Could you check a few things on this model? Use its own coordinates, in mm. A direction names the side the tool comes from. Round coordinates to 2 decimals unless told otherwise and drop trailing zeros. Loops run counter-clockwise (first coordinate to the right, second up) from the corner with the lowest first, then second, coordinate; pieces in that order, holes last. Notation, with made-up numbers: M -25,59.25 L 25,59.25 A31 ccw 25,98.25 Z; hole C 4,23 d11. An arc over 180 degrees is marked long. Answer in a Markdown table with one row per item.
```python
from build123d import *

# Parameters (mm, degrees)
SKETCH1_W        = 50
SKETCH1_H        = 50
SKETCH1_R        = 1.5
SUPPORT_DEPTH    = 8
NORTH_START      = -25
SKETCH2_W        = 20
SKETCH2_H        = 5
NORTH_CUT_DEPTH  = 4
WEST_START       = -25
SKETCH3_W        = 20
SKETCH3_H        = 5
WEST_CUT_DEPTH   = 4
EAST_START       = 25
SKETCH3_3_W      = 20
SKETCH3_3_H      = 5
EAST_DOWEL_DEPTH = 4


with BuildPart() as part:
    # Sketch1 → Support (new body)
    with BuildSketch(Plane(origin=(0, 0, 0), x_dir=(1, 0, 0), z_dir=(0, 1, 0))):
        Rectangle(SKETCH1_W, SKETCH1_H)
        with Locations(Location((-21, -21, 0), (0, 0, 270))):
            Circle(SKETCH1_R, mode=Mode.SUBTRACT)
        with Locations(Location((21, -21, 0), (0, 0, 270))):
            Circle(SKETCH1_R, mode=Mode.SUBTRACT)
        with BuildLine():
            Line((-13.031373033, 17.5), (17.5, 17.5))
            Line((17.5, 17.5), (17.5, -17.5))
            Line((17.5, -17.5), (-17.5, -17.5))
            Line((-17.5, -17.5), (-17.5, 13.031373033))
            ThreePointArc((-17.5, 13.031373033), (-20, 14.354248689), (-21, 17))
            Line((-21, 17), (-22.130136986, 20.01369863))
            ThreePointArc((-22.130136986, 20.01369863), (-22.060660172, 22.060660172), (-20.01369863, 22.130136986))
            Line((-20.01369863, 22.130136986), (-17, 21))
            ThreePointArc((-17, 21), (-14.354248689, 20), (-13.031373033, 17.5))
        make_face(mode=Mode.SUBTRACT)
        with Locations(Location((21, 21, 0), (0, 0, 270))):
            Circle(SKETCH1_R, mode=Mode.SUBTRACT)
    extrude(amount=SUPPORT_DEPTH)

    # Sketch2 → North Cut (cut)
    with BuildSketch(Plane.XY.offset(NORTH_START)):
        with Locations((0, 4)):
            Rectangle(SKETCH2_W, SKETCH2_H)
    extrude(amount=NORTH_CUT_DEPTH, mode=Mode.SUBTRACT)

    # Sketch3 → West Cut (cut)
    with BuildSketch(Plane(origin=(0, 0, 0), x_dir=(0, 0, -1), z_dir=(1, 0, 0)).offset(WEST_START)):
        with Locations((0, 4)):
            Rectangle(SKETCH3_W, SKETCH3_H)
    extrude(amount=WEST_CUT_DEPTH, mode=Mode.SUBTRACT)

    # Sketch3<3> → East Dowel (add)
    with BuildSketch(Plane(origin=(0, 0, 0), x_dir=(0, 0, -1), z_dir=(1, 0, 0)).offset(EAST_START)):
        with Locations((0, 4)):
            Rectangle(SKETCH3_3_W, SKETCH3_3_H)
    extrude(amount=EAST_DOWEL_DEPTH)


solid = part.part
```
1) I want a section at B-B, the plane x = 15. Please give me the cut outline in (y, z), plus the area to 3 significant figures.
Computed:
| item | result |
|---|---|
| outline | M 0,-25 L 8,-25 L 8,-17.5 L 0,-17.5 Z; M 0,17.5 L 8,17.5 L 8,25 L 0,25 Z |
| area | 120 mm² |
2) I want a section at C-C, the plane z = 21. Please give me the cut outline in (x, y), plus the area to 3 significant figures.
Computed:
| item | result |
|---|---|
| outline | M -25,0 L -22.5,0 L -22.5,8 L -25,8 Z; M -19.5,0 L 19.5,0 L 19.5,8 L -19.5,8 Z; M 22.5,0 L 25,0 L 25,8 L 22.5,8 Z |
| area | 352 mm² |
3) If we mould it in two halves opening along Y, with no side actions, what happens to faces 6 (the face through (-23, 6.5, 0)), 7 (the face through (-25, 7, 0)), 8 (the face through (27, 6.5, 0))? For each: released by +Y, released by -Y, zero draft, split by the parting line, or undercut.
Computed:
| item | result |
|---|---|
| face 6 | undercut |
| face 7 | zero draft |
| face 8 | released by +Y |
4) I want a section at D-D, the plane y = 3. Please give me the cut outline in (x, z), plus the area to 3 significant figures.
Computed:
| item | result |
|---|---|
| outline | M -25,-25 L -10,-25 L -10,-21 L 10,-21 L 10,-25 L 25,-25 L 25,-10 L 29,-10 L 29,10 L 25,10 L 25,25 L -25,25 L -25,10 L -21,10 L -21,-10 L -25,-10 Z; hole C -21,21 d3; hole M -22.13,-20.01 A1.5 ccw -20.01,-22.13 L -17,-21 A4 ccw -13.03,-17.5 L 17.5,-17.5 L 17.5,17.5 L -17.5,17.5 L -17.5,-13.03 A4 ccw -21,-17 Z; hole C 21,-21 d3; hole C 21,21 d3 |
| area | 1,130 mm² |
5) Which directions (+Z, -Z, +X, -X, +Y, -Y) give clear straight access to the entire face, cutting with the end or side of a thin tool? Please do faces 1 (the face through (27, 4, -10)), 2 (the face through (-18.528, 3.944, -21.573)), 3 (the face through (27, 4, 10)), 4 (the face through (-21, 4, 0)), 5 (the face through (0, 6.5, -23)).
Computed:
| item | result |
|---|---|
| face 1 | -Z, +X, +Y, -Y |
| face 2 | +Y, -Y |
| face 3 | +Z, +X, +Y, -Y |
| face 4 | -X |
| face 5 | -Z |
6) Will these pins go through, and if not, where does the flat tip stop? P1, Ø2.5, axis at y = 5, z = -4.5, coming from the -X side; P2, Ø2, axis at y = 4, z = -23, coming from the +X side; P3, Ø1.2, axis at x = 26.5, z = 1, coming from the +Y side; P4, Ø2.5, axis at x = -21, z = 21, coming from the +Y side.
Computed:
| item | result |
|---|---|
| P1 | stops at x = -21 |
| P2 | stops at x = 25 |
| P3 | stops at y = 6.5 |
| P4 | passes through |
7) I need wall thicknesses on line 1 (X direction, y = 4.5, z = 21); line 2 (X direction, y = 7.5, z = -12.5). Which ranges of each line are inside material? Lowest first, please.
Computed:
| item | result |
|---|---|
| line 1 | x = -25 to -22.5, -19.5 to 19.5, 22.5 to 25 |
| line 2 | x = -25 to -17.5, 17.5 to 25 |
8) I want a section at A-A, the plane z = 4. Please give me the cut outline in (x, y), plus the area to 3 significant figures.
Computed:
| item | result |
|---|---|
| outline | M -25,0 L -17.5,0 L -17.5,8 L -25,8 L -25,6.5 L -21,6.5 L -21,1.5 L -25,1.5 Z; M 17.5,0 L 25,0 L 25,1.5 L 29,1.5 L 29,6.5 L 25,6.5 L 25,8 L 17.5,8 Z |
| area | 120 mm² |
